from build123d import *

# Parameters (mm, degrees)
F0_W = 50
F0_H = 50
F2_R = 35.4285378843
F4_T = 1.8


# Not quite as in the source:
# - a shell that OpenCascade refuses in one call is made with other operations: the cavity is built on its own and cut out


with BuildPart() as f3:
    # F0 (on Top) → F3 section 0
    with BuildSketch(Plane.XY):
        Rectangle(F0_W, F0_H)
    # F2 (on offset) → F3 section 1
    with BuildSketch(Plane.XY.offset(30)):
        Circle(F2_R)
    loft()

    # F4: shell of thickness 1.8, made by hand


with BuildPart() as f4_core1:
    # F4_t2: copy of F3
    add(f3.part)

    # the walls: a layer under each face that stays
    f4_faces = [f4_core1.faces().sort_by_distance(p)[0] for p in [
        (0, 30.2142689408, 15),
        (-30.2142689408, 0, 15),
        (0, -30.2142689408, 15),
        (28.8658505055, -13.0289572392, 15),
        (28.8658505055, 13.0289572392, 15),
        (0, 0, 0),
    ]]
    thicken(f4_faces, amount=-F4_T, mode=Mode.SUBTRACT)


with BuildPart() as f3_1:
    add(f3.part)

    # what is left inside the walls is the cavity
    f4_cavity = [f4_core1.part.solids().sort_by_distance(p)[0] for p in [
        (0, -11.174295, 29.982),
    ]]
    add(f4_cavity, mode=Mode.SUBTRACT)


solid = f3_1.part
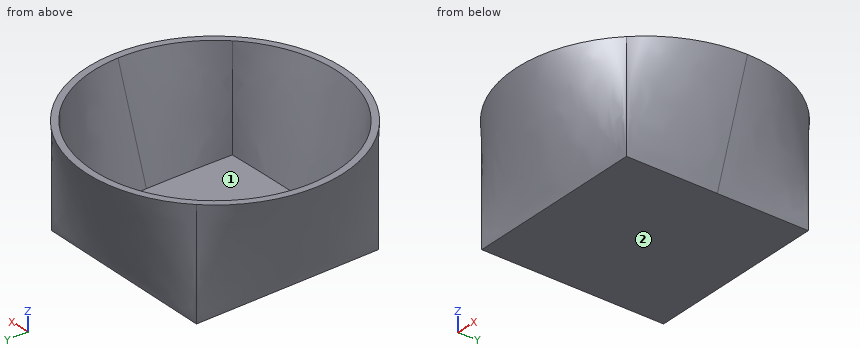
Work out the finished part from the listing and answer in its coordinate system (mm). Face numbers are marked on the shaded views. Give positions to 0.01 mm unless a question says otherwise; leave off trailing zeros. Answer as CSV lines item,"result". Start each with the question number.
Q1. Find the intervals of material crossed by L1, parallel to X at y = -21, z = 4.5; L2, parallel to Z at x = -8.5, y = 5.5; L3, parallel to X at y = -10, z = 15.5, in increasing order. Write a range as [from, to].
Q2. Given pin 1 Ø1.5 at (x, z) = (-5.5, 4) entering from -Y; pin 2 Ø10 at (x, z) = (-23, 9.5) entering from -Y; pin 3 Ø6 at (x, y) = (1, -14) entering from +Z, each flat-ended and moving along its own axis, determine where each tip first touches the part or whether it passes through.
Q3. The mould has two halves that part along X. Classify the marked faces 1 and 2: +X half, -X half, draft (parallel to the pull), parting line (faces both ways), or undercut.
Check result:
1,L1,"x = [-25.46, -23.64], [23.64, 25.46]"
1,L2,"z = [0, 1.8]"
1,L3,"x = [-29.57, -27.67], [27.67, 29.57]"
2,pin 1,"stops at y = -26.57"
2,pin 2,"stops at y = -26.9"
2,pin 3,"stops at z = 1.8"
3,face 1,"undercut"
3,face 2,"draft"
